Design review of the part built by this model. Coordinates are the model's own, in mm. Face numbers are marked on the shaded views. A direction names the side the tool comes from. Coordinates: 2 decimals unless noted, no trailing zeros. Loops run counter-clockwise (first coordinate to the right, second up) from the corner with the lowest first, then second, coordinate; pieces in that order, holes last. Notation, with made-up numbers: M 11.25,19 L 55.25,19 A27 ccw 55.25,48 Z; hole C 89.5,33.25 d9. An arc over 180 degrees is marked long. Put each result on its own line as item: value. Start each with the question number.
(1) Take a section at A-A, the plane x = 0. Give the boundary of the cut face in (y, z), then the cut area to 3 significant figures.
(2) Take a section at D-D, the plane z = -18. Give the boundary of the cut face in (x, y), then the cut area to 3 significant figures.
(3) Take a section at B-B, the plane z = 0. Give the boundary of the cut face in (x, y), then the cut area to 3 significant figures.
(4) The part is to be moulded in two halves that separate along Z. For the marked faces 3, 4 and 5, say which applies: +Z half, -Z half, draft (parallel to the pull), parting line (faces both ways), or undercut.
(5) For the marked faces 1 and 2, list the 3-axis set-ups (+Z, -Z, +X, -X, +Y, -Y) from which the entire face can be reached by the end or side of a thin tool; tool diameter is ignored.
(6) For probe 1 along Z at (x, y) = (12, -8.5); probe 2 along Z at (x, y) = (-3, -2); probe 3 along Z at (x, y) = (-8.5, -6.75), list the stretches that pass through material, from the lowest coordinate up. Write a range as [from, to].
(7) Take a section at C-C, the plane y = -1. Count the separate pieces of the cut face and the enclosed holes in it, then the cut area to 3 significant figures.
(8) Clearance check with flat-ended pins moving along their axes: pin 1 (2 mm diameter, centred on y = -3, z = -22, fed in from -X); pin 2 (6 mm diameter, centred on y = -2.5, z = 18, fed in from -X); pin 3 (4 mm diameter, centred on x = 10.5, y = -3, fed in from -Z). State where each tip first meets the part, or that it passes through.
```python
from build123d import *

# Parameters (mm, degrees)
SKETCH1_R             = 30
BOSS_EXTRUDE1_DEPTH   = 3
SKETCH2_R             = 23
BOSS_EXTRUDE2_DEPTH   = 1
SKETCH3_R             = 20
BOSS_EXTRUDE3_DEPTH   = 7
SKETCH12_R            = 10.5
CUT_EXTRUDE1_DEPTH    = 5
SKETCH16_R            = 6
CUT_EXTRUDE2_DEPTH    = 12
M3_TAPPED_HOLE1_D     = 2.5
M3_TAPPED_HOLE1_DEPTH = 29.248924226
M3_TAPPED_HOLE1_TIP   = 0.751075774


with BuildPart() as part:
    # Sketch1 → Boss-Extrude1 (new body)
    with BuildSketch(Plane(origin=(0, 0, 0), x_dir=(1, 0, 0), z_dir=(0, 1, 0))):
        Circle(SKETCH1_R)
    extrude(amount=-BOSS_EXTRUDE1_DEPTH)

    # Sketch2 → Boss-Extrude2 (add)
    with BuildSketch(Plane.XZ.offset(3)):
        Circle(SKETCH2_R)
    extrude(amount=BOSS_EXTRUDE2_DEPTH)

    # Sketch3 → Boss-Extrude3 (add)
    with BuildSketch(Plane.XZ.offset(4)):
        Circle(SKETCH3_R)
    extrude(amount=BOSS_EXTRUDE3_DEPTH)

    # Sketch12 → Cut-Extrude1 (cut)
    with BuildSketch(Plane.XZ.offset(11)):
        Circle(SKETCH12_R)
    extrude(amount=-CUT_EXTRUDE1_DEPTH, mode=Mode.SUBTRACT)

    # Sketch16 → Cut-Extrude2 (cut, through all)
    with BuildSketch(Plane(origin=(0, 0, 0), x_dir=(1, 0, 0), z_dir=(0, 1, 0))):
        Circle(SKETCH16_R)
    extrude(amount=-CUT_EXTRUDE2_DEPTH, mode=Mode.SUBTRACT)

    # M3 Tapped Hole1
    with Locations(Plane(origin=(0, 0, 0), x_dir=(1, 0, 0), z_dir=(0, 1, 0))):
        with Locations((-12.727922061, 12.727922061), (0, 18), (12.727922061, 12.727922061), (18, 0), (12.727922061, -12.727922061), (0, -18), (-12.727922061, -12.727922061), (-18, 0)):
            Hole(M3_TAPPED_HOLE1_D / 2, depth=M3_TAPPED_HOLE1_DEPTH)
            with Locations((0, 0, -(M3_TAPPED_HOLE1_DEPTH + M3_TAPPED_HOLE1_TIP / 2))):  # 118° drill point
                Cone(0, M3_TAPPED_HOLE1_D / 2, M3_TAPPED_HOLE1_TIP, mode=Mode.SUBTRACT)


solid = part.part
```
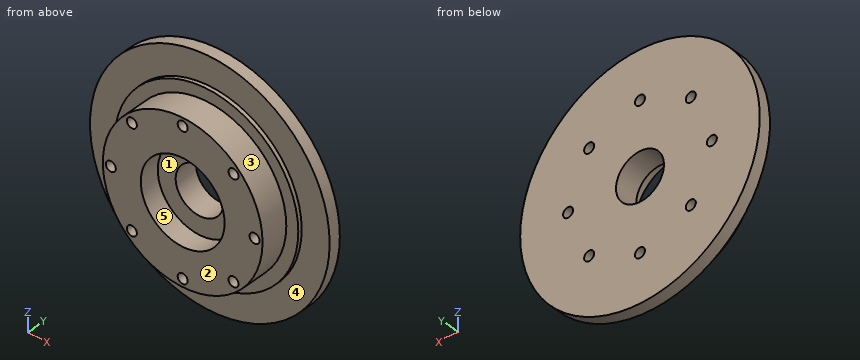
Computed values:
1. outline: M -11,-20 L -4,-20 L -4,-23 L -3,-23 L -3,-30 L 0,-30 L 0,-19.25 L -11,-19.25 Z; M -11,-16.75 L 0,-16.75 L 0,-6 L -6,-6 L -6,-10.5 L -11,-10.5 Z; M -11,10.5 L -6,10.5 L -6,6 L 0,6 L 0,16.75 L -11,16.75 Z; M -11,19.25 L 0,19.25 L 0,30 L -3,30 L -3,23 L -4,23 L -4,20 L -11,20 Z
1. area: 274 mm^2
2. outline: M -24,-3 L -14.32,-3 L -14.32,-4 L -8.72,-4 L -8.72,-11 L -1.25,-11 L -1.25,0 L -24,0 Z; M 1.25,-11 L 8.72,-11 L 8.72,-4 L 14.32,-4 L 14.32,-3 L 24,-3 L 24,0 L 1.25,0 Z
2. area: 267 mm^2
3. outline: M -30,-3 L -23,-3 L -23,-4 L -20,-4 L -20,-11 L -19.25,-11 L -19.25,0 L -30,0 Z; M -16.75,-11 L -10.5,-11 L -10.5,-6 L -6,-6 L -6,0 L -16.75,0 Z; M 6,-6 L 10.5,-6 L 10.5,-11 L 16.75,-11 L 16.75,0 L 6,0 Z; M 19.25,-11 L 20,-11 L 20,-4 L 23,-4 L 23,-3 L 30,-3 L 30,0 L 19.25,0 Z
3. area: 274 mm^2
4. face 3: parting line
4. face 4: draft
4. face 5: undercut
5. face 1: -Y
5. face 2: +Z, -Z, +X, -X, -Y
6. probe 1: z = [-16, -13.74], [-11.71, 11.71], [13.74, 16]
6. probe 2: z = [-29.85, -5.2], [5.2, 29.85]
6. probe 3: z = [-18.1, -6.16], [6.16, 18.1]
7. separate pieces: 1
7. enclosed holes: 9
7. area: 2,680 mm^2
8. pin 1: stops at x = -21.42
8. pin 2: stops at x = -25.98
8. pin 3: stops at z = -28.77
